Source: CAD feature listing. Evaluate the final solid. Frame: model axes, mm. A direction names the side the tool comes from. Give positions to 0.01 mm unless a question says otherwise; leave off trailing zeros. Loops run counter-clockwise (first coordinate to the right, second up) from the corner with the lowest first, then second, coordinate; pieces in that order, holes last. Notation, with made-up numbers: (7, 62.25) - (17, 62.25) arc R28 cw to (17, 84.25) - close; hole circle Ø10 at (71.25, 76.5). An arc over 180 degrees is marked (long way). Write each question's results on one line, items separated by ' | '. Start each with the question number.
(1) Material intervals for line 1 along X through (y, z) = (3.75, 62.5); line 2 along Z through (x, y) = (102.5, 2.5); line 3 along X through (y, z) = (5.25, -105), sorted ascending. Write a range as [from, to].
(2) Cut plane A-A on x = 93.5. Return the cut outline in (y, z).
(3) Pull-direction query (X, two-part tool) for faces 1 (the cylindrical face through (158.986, 3.498, 119.297)), 2 (the cylindrical face through (-133.986, 3.402, -94.297)), 3 (the flat face through (-2, 0, 109)), 4 (the cylindrical face through (-133.986, 3.402, 94.297)); classes: pulls with the +X half, pulls with the -X half, needs draft (parallel to the pull), parting line crosses it, or undercut.
(4) Reachability of faces 5 (the cylindrical face through (134.297, 3.402, -93.986)), 6 (the cylindrical face through (-159.297, 3.498, -118.986)) from +Z, -Z, +X, -X, +Y, -Y: full face, straight path, thin tool, end or side. Return the list, or none.
(5) Cut plane C-C on z = -7. Return the cut outline in (x, y).
(6) Cut plane B-B on y = 3.75. Give the number of separate pieces and of enclosed holes in the cut face, then the cut area to 3 significant figures.
(7) Contact query for a flat-ended pin moving along its axis: pin 1 (3.5 mm diameter, centred on x = 145, z = -105, fed in from +Y). Output: stop coordinate, or through.
from build123d import *

# Parameters (mm, degrees)
SKETCH1_W           = 330
SKETCH1_H           = 250
BOSS_EXTRUDE1_DEPTH = 6.9
SKETCH2_R           = 3
CUT_EXTRUDE1_DEPTH  = 7.9
SKETCH3_W           = 280
SKETCH3_H           = 200
CUT_EXTRUDE2_DEPTH  = 7.9
FILLET1_R           = 20
FILLET2_R           = 20
SKETCH4_R           = 3
CUT_EXTRUDE3_DEPTH  = 7.9


with BuildPart() as part:
    # Sketch1 → Boss-Extrude1 (new body)
    with BuildSketch(Plane(origin=(0, 0, 0), x_dir=(1, 0, 0), z_dir=(0, 1, 0))):
        Rectangle(SKETCH1_W, SKETCH1_H)
    extrude(amount=BOSS_EXTRUDE1_DEPTH)

    # Sketch2 → Cut-Extrude1 (cut, through all)
    with BuildSketch(Plane(origin=(0, 6.9, 0), x_dir=(1, 0, 0), z_dir=(0, 1, 0))):
        with Locations((-145, 105)):
            Circle(SKETCH2_R)
        with Locations((145, 105)):
            Circle(SKETCH2_R)
        with Locations((145, -105)):
            Circle(SKETCH2_R)
        with Locations((-145, -105)):
            Circle(SKETCH2_R)
    extrude(amount=-CUT_EXTRUDE1_DEPTH, mode=Mode.SUBTRACT)

    # Sketch3 → Cut-Extrude2 (cut, through all)
    with BuildSketch(Plane(origin=(0, 6.9, 0), x_dir=(1, 0, 0), z_dir=(0, 1, 0))):
        Rectangle(SKETCH3_W, SKETCH3_H)
    extrude(amount=-CUT_EXTRUDE2_DEPTH, mode=Mode.SUBTRACT)

    # Fillet1
    fillet1_edges = [part.edges().sort_by_distance(p)[0] for p in [
        (-165, 3.45, -125),
        (165, 3.45, -125),
        (165, 3.45, 125),
        (-165, 3.45, 125),
    ]]
    fillet(fillet1_edges, radius=FILLET1_R)

    # Fillet2
    fillet2_edges = [part.edges().sort_by_distance(p)[0] for p in [
        (-140, 3.45, 100),
        (-140, 3.45, -100),
        (140, 3.45, -100),
        (140, 3.45, 100),
    ]]
    fillet(fillet2_edges, radius=FILLET2_R)

    # Sketch4 → Cut-Extrude3 (cut, through all)
    with BuildSketch(Plane(origin=(0, 6.9, 0), x_dir=(1, 0, 0), z_dir=(0, 1, 0))):
        with Locations((-152.5, -62.5)):
            Circle(SKETCH4_R)
        with Locations((-102.5, -112.5)):
            Circle(SKETCH4_R)
        with Locations((102.5, -112.5)):
            Circle(SKETCH4_R)
        with Locations((152.5, -62.5)):
            Circle(SKETCH4_R)
        with Locations((152.5, 62.5)):
            Circle(SKETCH4_R)
        with Locations((102.5, 112.5)):
            Circle(SKETCH4_R)
        with Locations((-102.5, 112.5)):
            Circle(SKETCH4_R)
        with Locations((-152.5, 62.5)):
            Circle(SKETCH4_R)
    extrude(amount=-CUT_EXTRUDE3_DEPTH, mode=Mode.SUBTRACT)


solid = part.part
Ans:
1) line 1: [-165, -155.5], [-149.5, -140], [140, 149.5], [155.5, 165] | line 2: [-125, -115.5], [-109.5, -100], [100, 109.5], [115.5, 125] | line 3: [-165, -148], [-142, 142], [148, 165]
2) outline: (0, -125) - (6.9, -125) - (6.9, -100) - (0, -100) - close; (0, 100) - (6.9, 100) - (6.9, 125) - (0, 125) - close
3) face 1: pulls with the +X half | face 2: undercut | face 3: needs draft | face 4: undercut
4) face 5: +Y, -Y | face 6: -Z, -X, +Y, -Y
5) outline: (-165, 0) - (-140, 0) - (-140, 6.9) - (-165, 6.9) - close; (140, 0) - (165, 0) - (165, 6.9) - (140, 6.9) - close
6) separate pieces: 1 | enclosed holes: 13 | area: 26,200 mm^2
7) pin 1: through
